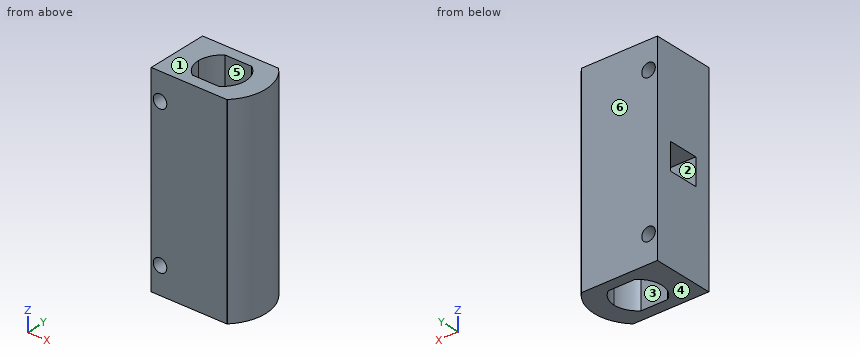
```python
from build123d import *

# Parameters (mm, degrees)
SALIENTE_EXTRUIR1_DEPTH = 52
CROQUIS3_W              = 0.615681901
CROQUIS3_H              = 16
SALIENTE_EXTRUIR2_DEPTH = 52
CROQUIS2_R              = 1.75
CORTAR_EXTRUIR1_DEPTH   = 52
SALIENTE_EXTRUIR3_START = -52
SALIENTE_EXTRUIR3_DEPTH = 52
CROQUIS4_W              = 6.89100463
CROQUIS4_H              = 7.9059588
CORTAR_EXTRUIR2_DEPTH   = 10


with BuildPart() as part:
    # Croquis1 → Saliente-Extruir1 (new body)
    with BuildSketch(Plane.XY):
        with BuildLine():
            Line((-3.032251305, 15.708802589), (-22.152251305, 15.708802589))
            Line((-22.152251305, 15.708802589), (-22.152251305, -0.291197411))
            Line((-22.152251305, -0.291197411), (-3.132125677, -0.291197411))
            ThreePointArc((-3.132125677, -0.291197411), (-3.082032439, -0.241353267), (-3.032251305, -0.191197411))
            ThreePointArc((-3.032251305, -0.191197411), (0.228795467, 7.758802589), (-3.032251305, 15.708802589))
        make_face()
        with BuildLine():
            Line((-15.641976571, 13.908802589), (-6.542526038, 13.908802589))
            ThreePointArc((-6.542526038, 13.908802589), (-3.442251305, 7.758802589), (-6.542526038, 1.608802589))
            Line((-6.542526038, 1.608802589), (-15.641976571, 1.608802589))
            ThreePointArc((-15.641976571, 1.608802589), (-18.742251305, 7.758802589), (-15.641976571, 13.908802589))
        make_face(mode=Mode.SUBTRACT)
    extrude(amount=SALIENTE_EXTRUIR1_DEPTH)

    # Croquis3 → Saliente-Extruir2 (add)
    with BuildSketch(Plane.XY.offset(52)):
        with Locations((-22.460092256, 7.708802589)):
            Rectangle(CROQUIS3_W, CROQUIS3_H)
    extrude(amount=-SALIENTE_EXTRUIR2_DEPTH)

    # Croquis2 → Cortar-Extruir1 (cut)
    with BuildSketch(Plane(origin=(0, 15.708802589, 0), x_dir=(1, 0, 0), z_dir=(0, 1, 0))):
        with Locations(Location((-20.467933206, -7, 0), (0, 0, 270))):
            Circle(CROQUIS2_R)
        with Locations(Location((-20.467933206, -45, 0), (0, 0, 270))):
            Circle(CROQUIS2_R)
    extrude(amount=-CORTAR_EXTRUIR1_DEPTH, mode=Mode.SUBTRACT)

    # Croquis5 → Saliente-Extruir3 (add)
    with BuildSketch(Plane.XY.offset(52).offset(SALIENTE_EXTRUIR3_START)):
        with BuildLine():
            ThreePointArc((-17.242251305, 7.758802589), (-16.52178307, 10.647173203), (-14.529183076, 12.858802589))
            Line((-14.529183076, 12.858802589), (-16.794224647, 12.858802589))
            ThreePointArc((-16.794224647, 12.858802589), (-17.024621708, 12.588862775), (-17.242251305, 12.308527855))
            Line((-17.242251305, 12.308527855), (-17.242251305, 7.758802589))
        make_face()
        with BuildLine():
            Line((-17.242251305, 3.209077323), (-17.242251305, 7.758802589))
            Line((-17.242251305, 7.758802589), (-17.242251305, 12.308527855))
            ThreePointArc((-17.242251305, 12.308527855), (-18.742251305, 7.758802589), (-17.242251305, 3.209077323))
        make_face()
        with BuildLine():
            Line((-16.794224647, 12.858802589), (-14.529183076, 12.858802589))
            ThreePointArc((-14.529183076, 12.858802589), (-12.889123587, 13.640447767), (-11.092251305, 13.908802589))
            Line((-11.092251305, 13.908802589), (-15.641976571, 13.908802589))
            ThreePointArc((-15.641976571, 13.908802589), (-16.244916255, 13.413229519), (-16.794224647, 12.858802589))
        make_face()
        with BuildLine():
            Line((-7.655319533, 12.858802589), (-5.390277962, 12.858802589))
            ThreePointArc((-5.390277962, 12.858802589), (-5.939586354, 13.413229519), (-6.542526038, 13.908802589))
            Line((-6.542526038, 13.908802589), (-11.092251305, 13.908802589))
            ThreePointArc((-11.092251305, 13.908802589), (-9.295379022, 13.640447767), (-7.655319533, 12.858802589))
        make_face()
        with BuildLine():
            ThreePointArc((-4.942251305, 12.308527855), (-5.159880902, 12.588862775), (-5.390277962, 12.858802589))
            Line((-5.390277962, 12.858802589), (-7.655319533, 12.858802589))
            ThreePointArc((-7.655319533, 12.858802589), (-5.662719539, 10.647173203), (-4.942251305, 7.758802589))
            Line((-4.942251305, 7.758802589), (-4.942251305, 12.308527855))
        make_face()
        with BuildLine():
            ThreePointArc((-3.442251305, 7.758802589), (-3.826922682, 10.154110502), (-4.942251305, 12.308527855))
            Line((-4.942251305, 12.308527855), (-4.942251305, 7.758802589))
            Line((-4.942251305, 7.758802589), (-4.942251305, 3.209077323))
            ThreePointArc((-4.942251305, 3.209077323), (-3.826922682, 5.363494676), (-3.442251305, 7.758802589))
        make_face()
        with BuildLine():
            Line((-4.942251305, 3.209077323), (-4.942251305, 7.758802589))
            ThreePointArc((-4.942251305, 7.758802589), (-5.662719539, 4.870431975), (-7.655319533, 2.658802589))
            Line((-7.655319533, 2.658802589), (-5.390277962, 2.658802589))
            ThreePointArc((-5.390277962, 2.658802589), (-5.159880902, 2.928742403), (-4.942251305, 3.209077323))
        make_face()
        with BuildLine():
            Line((-5.390277962, 2.658802589), (-7.655319533, 2.658802589))
            ThreePointArc((-7.655319533, 2.658802589), (-9.295379026, 1.87715741), (-11.092251313, 1.608802589))
            Line((-11.092251313, 1.608802589), (-6.542526038, 1.608802589))
            ThreePointArc((-6.542526038, 1.608802589), (-5.939586354, 2.104375659), (-5.390277962, 2.658802589))
        make_face()
        with BuildLine():
            ThreePointArc((-11.092251313, 1.608802589), (-9.295379026, 1.87715741), (-7.655319533, 2.658802589))
            Line((-7.655319533, 2.658802589), (-14.529183076, 2.658802589))
            ThreePointArc((-14.529183076, 2.658802589), (-12.889123591, 1.877157412), (-11.092251313, 1.608802589))
        make_face()
        with BuildLine():
            ThreePointArc((-11.092251313, 1.608802589), (-12.889123591, 1.877157412), (-14.529183076, 2.658802589))
            Line((-14.529183076, 2.658802589), (-16.794224647, 2.658802589))
            ThreePointArc((-16.794224647, 2.658802589), (-16.244916255, 2.104375659), (-15.641976571, 1.608802589))
            Line((-15.641976571, 1.608802589), (-11.092251313, 1.608802589))
        make_face()
        with BuildLine():
            ThreePointArc((-14.529183076, 2.658802589), (-16.52178307, 4.870431975), (-17.242251305, 7.758802589))
            Line((-17.242251305, 7.758802589), (-17.242251305, 3.209077323))
            ThreePointArc((-17.242251305, 3.209077323), (-17.024621708, 2.928742403), (-16.794224647, 2.658802589))
            Line((-16.794224647, 2.658802589), (-14.529183076, 2.658802589))
        make_face()
        with BuildLine():
            Line((-6.542526038, 1.608802589), (-11.092251313, 1.608802589))
            Line((-11.092251313, 1.608802589), (-15.641976571, 1.608802589))
            ThreePointArc((-15.641976571, 1.608802589), (-11.092251305, 0.108802589), (-6.542526038, 1.608802589))
        make_face()
        with BuildLine():
            Line((-11.092251305, 13.908802589), (-6.542526038, 13.908802589))
            ThreePointArc((-6.542526038, 13.908802589), (-11.092251305, 15.408802589), (-15.641976571, 13.908802589))
            Line((-15.641976571, 13.908802589), (-11.092251305, 13.908802589))
        make_face()
        with BuildLine():
            Line((-14.529183076, 12.858802589), (-7.655319533, 12.858802589))
            ThreePointArc((-7.655319533, 12.858802589), (-9.295379022, 13.640447767), (-11.092251305, 13.908802589))
            ThreePointArc((-11.092251305, 13.908802589), (-12.889123587, 13.640447767), (-14.529183076, 12.858802589))
        make_face()
    extrude(amount=SALIENTE_EXTRUIR3_DEPTH)

    # Croquis4 → Cortar-Extruir2 (cut)
    with BuildSketch(Plane.ZY.offset(22.767933206)):
        with Locations((26, 7.708802589)):
            Rectangle(CROQUIS4_W, CROQUIS4_H)
    extrude(amount=-CORTAR_EXTRUIR2_DEPTH, mode=Mode.SUBTRACT)


solid = part.part
```
The model under review builds one solid part; all positions refer to its coordinate system, in mm. Face numbers are marked on the shaded views. A direction names the side the tool comes from. Give positions to 0.01 mm unless a question says otherwise; leave off trailing zeros. Write each loop counter-clockwise with the first axis right and the second up, starting at its lowest first coordinate (ties: lowest second). Pieces come first, ordered by that corner, then holes. Notation, with made-up numbers: M 63,76.25 L 115,76.25 A21 ccw 115,113.25 Z; hole C 58,-33.5 d5. An arc over 180 degrees is marked long. Write item = value, one per line. Start each with the question number.
Q1. We need section B-B (x = -14). State the section outline as (y, z) points.
Q2. Machinability: for the marked faces 5 and 6, which of the approach directions +Z, -Z, +X, -X, +Y, -Y give a long, thin tool a straight path to every point of the face, cutting with its end or side? Answer none if there is none.
Q3. Mouldability with a two-part tool opening along Z and no side actions: class the marked faces 1, 2, 3 and 4 as released by +Z, released by -Z, zero draft, split by the parting line, or undercut.
Q4. Clearance check with a flat-ended pin moving along its axis: pin 1 (3 mm diameter, centred on x = -20.47, z = 7, fed in from +Y). State where the tip first meets the part, or that it passes through.
Q5. We need section A-A (y = 4.75). State the section outline as (x, z) points.
Q6. For line 1 (X direction, y = 3, z = 45); line 2 (Y direction, x = -8, z = 47.5); line 3 (Z direction, x = -20, y = 1), list the stretches that pass through material, from the lowest coordinate up.
Q7. We need section D-D (y = 9.75). State the section outline as (x, z) points, plus the area to 3 significant figures.
Q8. We need section C-C (z = 46). State the section outline as (x, y) points.
Result set:
q1.outline = M -0.29,0 L 2.66,0 L 2.66,52 L -0.29,52 Z; M 12.86,0 L 15.71,0 L 15.71,52 L 12.86,52 Z
q2.face_5 = +Z, -Z
q2.face_6 = +Z, -Z, +X, -X, +Y
q3.face_1 = released by +Z
q3.face_2 = undercut
q3.face_3 = zero draft
q3.face_4 = released by -Z
q4.pin_1 = through
q5.outline = M -22.77,0 L -16.46,0 L -16.46,22.55 L -22.77,22.55 Z; M -22.77,29.45 L -16.46,29.45 L -16.46,52 L -22.77,52 Z; M -5.73,0 L -0.18,0 L -0.18,52 L -5.73,52 Z; hole C -20.47,7 d3.5; hole C -20.47,45 d3.5
q6.line_1 = -22.77 to -22.22, -18.72 to -14.99, -7.2 to -0.82
q6.line_2 = -0.29 to 2.66, 12.86 to 15.71
q6.line_3 = 0 to 5.31, 8.69 to 43.31, 46.69 to 52
q7.outline = M -22.77,0 L -16.91,0 L -16.91,22.55 L -22.77,22.55 Z; M -22.77,29.45 L -16.91,29.45 L -16.91,52 L -22.77,52 Z; M -5.27,0 L 0.05,0 L 0.05,52 L -5.27,52 Z; hole C -20.47,7 d3.5; hole C -20.47,45 d3.5
q7.area = 522 mm2
q8.outline = M -22.77,-0.29 L -21.9,-0.29 L -21.9,15.71 L -22.77,15.71 Z; M -19.03,-0.29 L -3.13,-0.29 A11.32 ccw -3.03,-0.19 A11.32 ccw -3.03,15.71 L -19.03,15.71 Z; hole M -14.53,2.66 L -7.66,2.66 A6.15 ccw -7.66,12.86 L -14.53,12.86 A6.15 ccw Z
